```python
from build123d import *

# Parameters (mm, degrees)
F1_DEPTH = 6.35


with BuildPart() as f1:
    # F0 (on Front) → F1 (new body)
    with BuildSketch(Plane.XZ):
        with BuildLine():
            ThreePointArc((-37.2364, 0), (-33.992783, 7.830783), (-26.162, 11.0744))
            Line((-26.162, 11.0744), (-26.162, 20.32))
            ThreePointArc((-26.162, 20.32), (-39.471894, 13.309894), (-46.482, 0))
            Line((-46.482, 0), (-37.2364, 0))
        make_face()
        with BuildLine():
            ThreePointArc((-46.482, -7.0612), (-34.50328, -10.90329), (-26.162, -20.32))
            Line((-26.162, -20.32), (-26.162, -11.0744))
            ThreePointArc((-26.162, -11.0744), (-33.992783, -7.830783), (-37.2364, 0))
            Line((-37.2364, 0), (-46.482, 0))
            Line((-46.482, 0), (-46.482, -7.0612))
        make_face()
        with BuildLine():
            Line((0, -17.78), (0, -11.0744))
            ThreePointArc((0, -11.0744), (-7.830783, -7.830783), (-11.0744, 0))
            Line((-11.0744, 0), (-15.0876, 0))
            ThreePointArc((-15.0876, 0), (-18.331217, -7.830783), (-26.162, -11.0744))
            Line((-26.162, -11.0744), (-26.162, -20.32))
            ThreePointArc((-26.162, -20.32), (-13.808095, -11.56092), (0, -17.78))
        make_face()
        with BuildLine():
            Line((15.0876, 0), (11.0744, 0))
            ThreePointArc((11.0744, 0), (7.830783, -7.830783), (0, -11.0744))
            Line((0, -11.0744), (0, -17.78))
            ThreePointArc((0, -17.78), (13.808095, -11.56092), (26.162, -20.32))
            Line((26.162, -20.32), (26.162, -11.0744))
            ThreePointArc((26.162, -11.0744), (18.331217, -7.830783), (15.0876, 0))
        make_face()
        with BuildLine():
            ThreePointArc((37.2364, 0), (33.992783, -7.830783), (26.162, -11.0744))
            Line((26.162, -11.0744), (26.162, -20.32))
            ThreePointArc((26.162, -20.32), (34.50328, -10.90329), (46.482, -7.0612))
            Line((46.482, -7.0612), (46.482, 0))
            Line((46.482, 0), (37.2364, 0))
        make_face()
        with BuildLine():
            Line((26.162, 20.32), (26.162, 11.0744))
            ThreePointArc((26.162, 11.0744), (33.992783, 7.830783), (37.2364, 0))
            Line((37.2364, 0), (46.482, 0))
            ThreePointArc((46.482, 0), (39.471894, 13.309894), (26.162, 20.32))
        make_face()
        with BuildLine():
            ThreePointArc((0, 11.0744), (7.830783, 7.830783), (11.0744, 0))
            Line((11.0744, 0), (15.0876, 0))
            ThreePointArc((15.0876, 0), (18.331217, 7.830783), (26.162, 11.0744))
            Line((26.162, 11.0744), (26.162, 20.32))
            ThreePointArc((26.162, 20.32), (15.737544, 12.305846), (4.953, 19.828449))
            ThreePointArc((4.953, 19.828449), (4.954587, 19.703036), (4.953, 19.577624))
            Line((4.953, 19.577624), (4.953, 14.748449))
            Line((4.953, 14.748449), (0, 14.748449))
            Line((0, 14.748449), (0, 11.0744))
        make_face()
        with BuildLine():
            ThreePointArc((-11.0744, 0), (-7.830783, 7.830783), (0, 11.0744))
            Line((0, 11.0744), (0, 14.748449))
            Line((0, 14.748449), (-4.953, 14.748449))
            Line((-4.953, 14.748449), (-4.953, 19.577624))
            ThreePointArc((-4.953, 19.577624), (-4.954587, 19.703036), (-4.953, 19.828449))
            ThreePointArc((-4.953, 19.828449), (-15.737544, 12.305846), (-26.162, 20.32))
            Line((-26.162, 20.32), (-26.162, 11.0744))
            ThreePointArc((-26.162, 11.0744), (-18.331217, 7.830783), (-15.0876, 0))
            Line((-15.0876, 0), (-11.0744, 0))
        make_face()
        with BuildLine():
            Line((-4.953, 14.748449), (0, 14.748449))
            ThreePointArc((0, 14.748449), (-3.458798, 16.155551), (-4.953, 19.577624))
            Line((-4.953, 19.577624), (-4.953, 14.748449))
        make_face()
        with BuildLine():
            ThreePointArc((4.953, 19.577624), (3.458798, 16.155551), (0, 14.748449))
            Line((0, 14.748449), (4.953, 14.748449))
            Line((4.953, 14.748449), (4.953, 19.577624))
        make_face()
    extrude(amount=F1_DEPTH)


solid = f1.part
```
Part model, mm, in its own coordinate system. Give positions to 0.01 mm unless a question says otherwise; leave off trailing zeros. Order: outer loops, then holes, each group sorted by start corner. A loop starts at its lowest first (then second) coordinate and runs counter-clockwise, first axis right, second up. Notation, with made-up numbers: M 7,52.5 L 39,52.5 A36 cw 39,90.5 Z; hole C 8.25,-24.75 d10. An arc over 180 degrees is marked long. Use a Markdown table: item, result. Add a question column.
(1) Saw through at B-B, the plane y = -4.25. Give the cut face in (x, z), and give its area (3 significant figures).
(2) Saw through at A-A, the plane x = -22.5. Give the cut face in (y, z), and give its area (3 significant figures).
(3) Mould opens along X. For faces 1 (the face through (34.354, -3.131, -11.001)), 2 (the face through (13.59, -3.13, -11.54)), 3 (the face through (15.93, -3.13, 12.31)), 4 (the face through (-46.482, -3, -3)) say: +X half, -X half, draft (parallel to the pull), parting line (faces both ways), or undercut.
(4) Saw through at D-D, the plane z = -13. Give the cut face in (x, y).
(5) Probe line 1 along X through (y, z) = (-5, -6); line 2 along X through (y, z) = (-5.25, -17); line 3 along X through (y, z) = (-3.5, -1). List the from-to ranges inside material, lowest first. Write a range as [from, to].
(6) Drop flat-ended pins along their axis: P1, Ø3, axis at x = -21, y = -1, coming from the +Z side; P2, Ø3, axis at y = -3, z = 13.5, coming from the +X side. Give the stop position or say it passes through.
(7) Saw through at C-C, the plane z = 5. Give the cut face in (x, y), and give its area (3 significant figures).
Answer key:
| question | item | result |
|---|---|---|
| 1 | outline | M -46.48,-7.06 A23.77 cw -26.16,-20.32 A15.24 cw 0,-17.78 A15.24 cw 26.16,-20.32 A23.77 cw 46.48,-7.06 L 46.48,0 A25.4 ccw 26.16,20.32 A11.13 cw 4.95,19.83 A4.96 cw 4.95,19.58 A4.95 cw -4.95,19.58 A4.96 cw -4.95,19.83 A11.13 cw -26.16,20.32 A25.4 ccw -46.48,0 Z; hole M -37.24,0 A11.07 ccw -26.16,-11.07 A11.07 ccw -15.09,0 A11.07 ccw -26.16,11.07 A11.07 ccw Z; hole M -11.07,0 A11.07 ccw 0,-11.07 A11.07 ccw 11.07,0 A11.07 ccw 0,11.07 A11.07 ccw Z; hole M 15.09,0 A11.07 ccw 26.16,-11.07 A11.07 ccw 37.24,0 A11.07 ccw 26.16,11.07 A11.07 ccw Z |
| 1 | area | 1,360 mm^2 |
| 2 | outline | M -6.35,-15.37 L 0,-15.37 L 0,-10.45 L -6.35,-10.45 Z; M -6.35,10.45 L 0,10.45 L 0,14.8 L -6.35,14.8 Z |
| 2 | area | 58.9 mm^2 |
| 3 | face 1 | +X half |
| 3 | face 2 | undercut |
| 3 | face 3 | undercut |
| 3 | face 4 | -X half |
| 4 | outline | M -31.75,-6.35 L -18.95,-6.35 L -18.95,0 L -31.75,0 Z; M -5.72,-6.35 L 5.72,-6.35 L 5.72,0 L -5.72,0 Z; M 18.95,-6.35 L 31.75,-6.35 L 31.75,0 L 18.95,0 Z |
| 5 | line 1 | [-46.48, -35.47], [-16.85, -9.31], [9.31, 16.85], [35.47, 46.48] |
| 5 | line 2 | [-28.15, -24.07], [-0.61, 0.61], [24.07, 28.15] |
| 5 | line 3 | [-46.48, -37.19], [-15.13, -11.03], [11.03, 15.13], [37.19, 46.48] |
| 6 | P1 | z = 14.8 |
| 6 | P2 | x = 40.69 |
| 7 | outline | M -45.01,-6.35 L -36.04,-6.35 L -36.04,0 L -45.01,0 Z; M -16.28,-6.35 L -9.88,-6.35 L -9.88,0 L -16.28,0 Z; M 9.88,-6.35 L 16.28,-6.35 L 16.28,0 L 9.88,0 Z; M 36.04,-6.35 L 45.01,-6.35 L 45.01,0 L 36.04,0 Z |
| 7 | area | 195 mm^2 |
